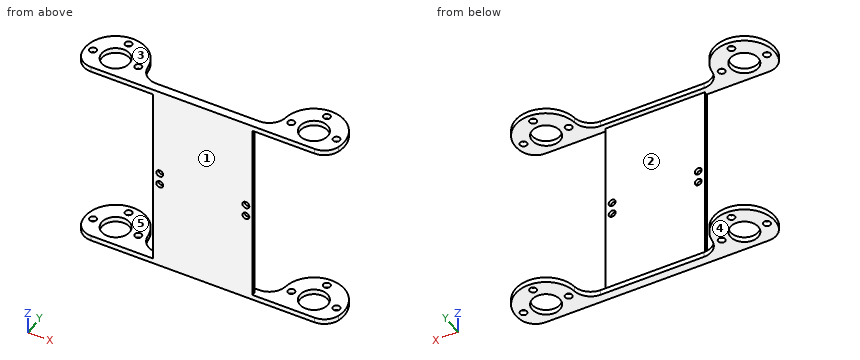
Autodesk Inventor part; units mm, degrees
ref_plane "YZ Plane" through (0, 0, 0) normal (1, 0, 0) x (0, 1, 0)
ref_plane "XZ Plane" through (0, 0, 0) normal (0, 1, 0) x (-1, 0, 0)
ref_plane "XY Plane" through (0, 0, 0) normal (0, 0, 1) x (1, 0, 0)
sketch "Main Body Sketch" plane through (0, 0, 0) normal (0, 1, 0) x (-1, 0, 0)
  line L0 (-28.5, -56.15) -> (28.5, -56.15)
  line L1 (28.5, -56.15) -> (28.5, 56.15)
  line L2 (28.5, 56.15) -> (-28.5, 56.15)
  line L3 (-28.5, 56.15) -> (-28.5, -56.15)
  line L4 (-28.5, -56.15) -> (28.5, 56.15) construction
  line L5 (28.5, -56.15) -> (-28.5, 56.15) construction
  line L6 (0, 46.8487) -> (0, -109.4037) construction
  circle A0 centre (-24.75, 3.5) radius 2
  circle A1 centre (24.75, 3.5) radius 2
  circle A2 centre (24.75, -3.5) radius 2
  circle A3 centre (-24.75, -3.5) radius 2
  point P0 (0, 0)
  dimension "d0" = 57
  dimension "d1" = 112.3
  dimension "d2" = 4
  dimension "d3" = 24.75
  dimension "d4" = 52.65
  dimension "d7" = 7
  dimension "d34" = 52.65
  dimension "d35" = 3.75
  dimension "d36" = 3.75
  dimension "d37" = 3.75
  dimension "d38" = 52.65
extrude "Main Body Extrusion" add sketch "Main Body Sketch" along normal blind 2
sketch "Mounting Circles" plane through (-28.5, 0, 56.15) normal (0, 0, 1) x (1, 0, 0)
  circle A0 centre (-28.5, 12) radius 8
  arc A1 (-12.457, 5.0091) -> (-41.2377, 0) centre (-28.5, 12) ccw
  line L0 (-12.457, 5.0091) -> (0, 5.0091)
  line L1 (28.5, -10.7409) -> (28.5, 31.3182) construction
  circle A2 centre (-28.5, 25) radius 2
  circle A3 centre (-41.5, 12) radius 2
  circle A4 centre (-15.5, 12) radius 2
  circle A5 centre (85.5, 12) radius 8
  arc A6 (98.2377, 0) -> (69.457, 5.0091) centre (85.5, 12) ccw
  line L2 (69.457, 5.0091) -> (57, 5.0091)
  line L3 (57, 0) -> (57, 2) construction
  circle A7 centre (85.5, 25) radius 2
  circle A8 centre (98.5, 12) radius 2
  circle A9 centre (72.5, 12) radius 2
  line L4 (0, 5.0091) -> (57, 5.0091)
  line L5 (0, 0) -> (0, 2) construction
  line L6 (57, 0) -> (0, 0) construction
  line L7 (-41.2377, 0) -> (98.2377, 0)
  point P0 (28.5, 0)
  dimension "d10" = 57
  dimension "d11" = 16
  dimension "d13" = 35
  dimension "d19" = 4
  dimension "d20" = 4
  dimension "d21" = 4
  dimension "d22" = 13
  dimension "d23" = 13
  dimension "d24" = 13
  dimension "d33" = 114
extrude "Side Attatchments" add sketch "Mounting Circles" against normal blind 3
fillet "Fillet5" radius 10 2 edges at (-40.957, 5.0091, 54.65) (40.957, 5.0091, 54.65)
fillet "Fillet6" radius 10 2 edges at (-69.7377, 0, 54.65) (69.7377, 0, 54.65)
mirror "Mirror1" about plane through (0, 0, 0) normal (0, 0, 1) of "Side Attatchments"
fillet "Fillet7" radius 10 4 edges at (-40.957, 5.0091, -54.65) (40.957, 5.0091, -54.65) (-69.7377, 0, -54.65) (69.7377, 0, -54.65)
ref_plane "Work Plane1" through (0, 0, 0) normal (0, 0, 1) x (1, 0, 0)
properties part number "Servo Plate V3"
Read the model definition and answer for the solid it produces. Units are mm, in the model's axes. Face numbers are marked on the shaded views. A direction names the side the tool comes from. Round coordinates to 2 decimals unless told otherwise and drop trailing zeros. Write each loop counter-clockwise with the first axis right and the second up, starting at its lowest first coordinate (ties: lowest second). Pieces come first, ordered by that corner, then holes. Notation, with made-up numbers: (14.25, -7.5) -> (46.25, -7.5) arc R27 cw to (46.25, 9.5) -> close; hole circle Ø8 at (-2, 34). An arc over 180 degrees is marked (long way). Answer in a Markdown table with one row per item. Add a question column.
1) Find section C-C, the plane y = 25. State how many separate pieces and enclosed holes the cut face has, and give its area (3 significant figures).
2) Find section A-A, the plane x = 57. Determine the outline of the cut face in (y, z).
3) Which of the six approach directions +Z, -Z, +X, -X, +Y, -Y give full straight-line access (tool end or side, diameter ignored) to the marked faces 1 and 2?
4) Find section D-D, the plane x = -24.75. Determine the outline of the cut face in (y, z).
5) Given P1, Ø1.5, axis at x = 4, z = 55, coming from the +Y side; P2, Ø14.5, axis at x = 57, y = 12, coming from the +Z side; P3, Ø5, axis at x = -23.5, z = 27, coming from the +Y side, each flat-ended and moving along its own axis, determine where each tip first touches the part or whether it passes through.
6) Consider line 1 (Y direction, x = 57, z = -53.8); line 2 (Z direction, x = -16, y = 4.5); line 3 (Y direction, x = -26.5, z = 17.5). Determine where each line is inside the solid, lowest interval first.
7) Find section B-B, the plane z = 3.5. Determine the outline of the cut face in (x, y), and give its area (3 significant figures).
8) Determine the mould class of the marked faces 3, 4 and 5 for opening direction Z: pulls with the +Z half, pulls with the -Z half, needs draft (parallel to the pull), parting line crosses it, or undercut.
Findings below:
| question | item | result |
|---|---|---|
| 1 | separate pieces | 8 |
| 1 | enclosed holes | 0 |
| 1 | area | 233 mm² |
| 2 | outline | (0, -56.15) -> (4, -56.15) -> (4, -53.15) -> (0, -53.15) -> close; (0, 53.15) -> (4, 53.15) -> (4, 56.15) -> (0, 56.15) -> close; (20, -56.15) -> (23, -56.15) -> (23, -53.15) -> (20, -53.15) -> close; (20, 53.15) -> (23, 53.15) -> (23, 56.15) -> (20, 56.15) -> close; (27, -56.15) -> (29.5, -56.15) -> (29.5, -53.15) -> (27, -53.15) -> close; (27, 53.15) -> (29.5, 53.15) -> (29.5, 56.15) -> (27, 56.15) -> close |
| 3 | face 1 | +Z, -Z, +X, -X, -Y |
| 3 | face 2 | +X, -X, +Y |
| 4 | outline | (0, -56.15) -> (5.01, -56.15) -> (5.01, -53.15) -> (2, -53.15) -> (2, -5.5) -> (0, -5.5) -> close; (0, -1.5) -> (2, -1.5) -> (2, 1.5) -> (0, 1.5) -> close; (0, 5.5) -> (2, 5.5) -> (2, 53.15) -> (5.01, 53.15) -> (5.01, 56.15) -> (0, 56.15) -> close |
| 5 | P1 | y = 5.01 |
| 5 | P2 | through |
| 5 | P3 | y = 2 |
| 6 | line 1 | 0 to 4, 20 to 23, 27 to 29.5 |
| 6 | line 2 | -56.15 to -53.15, 53.15 to 56.15 |
| 6 | line 3 | 0 to 2 |
| 7 | outline | (-28.5, 0) -> (-26.75, 0) -> (-26.75, 2) -> (-28.5, 2) -> close; (-22.75, 0) -> (22.75, 0) -> (22.75, 2) -> (-22.75, 2) -> close; (26.75, 0) -> (28.5, 0) -> (28.5, 2) -> (26.75, 2) -> close |
| 7 | area | 98.0 mm² |
| 8 | face 3 | pulls with the +Z half |
| 8 | face 4 | pulls with the -Z half |
| 8 | face 5 | undercut |
